Source: CAD feature listing. Evaluate the final solid. Frame: model axes, mm. Give positions to 0.01 mm unless a question says otherwise; leave off trailing zeros. Loops run counter-clockwise (first coordinate to the right, second up) from the corner with the lowest first, then second, coordinate; pieces in that order, holes last. Notation, with made-up numbers: M 26,0.5 L 31,0.5 A3 ccw 31,4.5 Z; hole C 11,-17.75 d3. An arc over 180 degrees is marked long. Put each result on its own line as item: value. Start each with the question number.
```python
from build123d import *

# Parameters (mm, degrees)
BOSS_EXTRUDE1_DEPTH = 25


with BuildPart() as part:
    # Sketch1 → Boss-Extrude1 (new body)
    with BuildSketch(Plane.XY):
        Polygon((0, 0), (100, 0), (100, 17.571317314), (60, 45.579618843), (0, 35), align=None)
    extrude(amount=BOSS_EXTRUDE1_DEPTH)


solid = part.part
```
1. Section A-A, the plane z = 2.5. Output: boundary loops of the cut face in (x, y).
2. Section B-B, the plane x = 21.5. Output: boundary loops of the cut face in (y, z), plus the area to 3 significant figures.
3. Ray query, line 1 (Y direction, x = 33, z = 18.25); line 2 (Y direction, x = 94, z = 7.75); line 3 (X direction, y = 19.5, z = 22). Return the intervals inside material, ascending.
4. Section C-C, the plane y = 33. Output: boundary loops of the cut face in (x, z), plus the area to 3 significant figures.
Results found:
1. outline: M 0,0 L 100,0 L 100,17.57 L 60,45.58 L 0,35 Z
2. outline: M 0,0 L 38.79,0 L 38.79,25 L 0,25 Z
2. area: 970 mm²
3. line 1: 0 to 40.82
3. line 2: 0 to 21.77
3. line 3: 0 to 97.25
4. outline: M 0,0 L 77.97,0 L 77.97,25 L 0,25 Z
4. area: 1,950 mm²
